```python
from build123d import *

# Parameters (mm, degrees)
CROQUIS1_R              = 0.5
SALIENTE_EXTRUIR1_DEPTH = 3
MATRIZC1_COUNT          = 2
CROQUIS2_R              = 4
CROQUIS2_R_2            = 3
SALIENTE_EXTRUIR2_DEPTH = 2
CHAFL_N1_SIZE           = 1
CHAFL_N1_SIZE2          = 0.577350269


with BuildPart() as part:
    # Croquis1 → Saliente-Extruir1 (new body)
    with BuildSketch(Plane(origin=(0, 0, 0), x_dir=(1, 0, 0), z_dir=(0, 1, 0))):
        with BuildLine():
            Line((-4, 0), (-4, 6.574293681))
            ThreePointArc((-4, 6.574293681), (-3.974394349, 6.996885575), (-3.897952052, 7.413294188))
            Line((-3.897952052, 7.413294188), (-1.698976026, 16.319147094))
            ThreePointArc((-1.698976026, 16.319147094), (0, 17.649646841), (1.698976026, 16.319147094))
            Line((1.698976026, 16.319147094), (3.897952052, 7.413294188))
            ThreePointArc((3.897952052, 7.413294188), (3.974394349, 6.996885575), (4, 6.574293681))
            Line((4, 6.574293681), (4, 0))
            Line((4, 0), (1.25, 0))
            ThreePointArc((1.25, 0), (0, 1.25), (-1.25, 0))
            Line((-1.25, 0), (-4, 0))
        make_face()
        with Locations((0, 15.899646841)):
            Circle(CROQUIS1_R, mode=Mode.SUBTRACT)
        with Locations((0, 12.899646841)):
            Circle(CROQUIS1_R, mode=Mode.SUBTRACT)
        with Locations((0, 9.899646841)):
            Circle(CROQUIS1_R, mode=Mode.SUBTRACT)
        with Locations((0, 6.899646841)):
            Circle(CROQUIS1_R, mode=Mode.SUBTRACT)
    saliente_extruir1 = extrude(amount=SALIENTE_EXTRUIR1_DEPTH)

    # MatrizC1: Saliente-Extruir1 ×2 about axis
    matrizc1_axis = Axis((0, 0, 0), (0, 1, 0))
    for i in range(1, MATRIZC1_COUNT):
        add(saliente_extruir1.rotate(matrizc1_axis, i * 360 / MATRIZC1_COUNT))

    # Croquis2 → Saliente-Extruir2 (add)
    with BuildSketch(Plane(origin=(0, 3, 0), x_dir=(1, 0, 0), z_dir=(0, 1, 0))):
        Circle(CROQUIS2_R)
        Circle(CROQUIS2_R_2, mode=Mode.SUBTRACT)
    extrude(amount=SALIENTE_EXTRUIR2_DEPTH)

    # Chaflán1
    chafl_n1_edges = [part.edges().sort_by_distance(p)[0] for p in [
        (-4, 5, 0),
    ]]
    chafl_n1_side = [part.faces().sort_by_distance(p)[0] for p in [
        (-4, 4, 0),
    ]]
    chamfer(chafl_n1_edges, length=CHAFL_N1_SIZE, length2=CHAFL_N1_SIZE2, reference=chafl_n1_side[0])


solid = part.part
```
Could you check a few things on this model? Use its own coordinates, in mm. A direction names the side the tool comes from. Round coordinates to 2 decimals unless told otherwise and drop trailing zeros. Loops run counter-clockwise (first coordinate to the right, second up) from the corner with the lowest first, then second, coordinate; pieces in that order, holes last.
Q1. I want a section at A-A (y = 2.25). Give the number of separate pieces and of enclosed holes in the cut face, and give its area (3 significant figures).
Q2. Please list where these lines run through material, in increasing order: L1, parallel to Z at x = 0, y = 3.85; L2, parallel to Y at x = -1.75, z = -7; L3, parallel to Z at x = -1, y = 3.2.
Q3. On a 3-axis mill with a long thin cutter (end or side, diameter ignored), from which of +Z, -Z, +X, -X, +Y, -Y can I reach the whole of each face in a straight line? I mean faces 1 (the flat face through (1, 3, -1)), 2 (the flat face through (4, 1, 0)). Say none if no direction works.
Q4. I want a section at D-D (z = -14). Write out the boundary of the cut face in (x, y), and give its area (3 significant figures).
Q5. Thinking about a two-plate mould opening in X: for faces 3 (the cylindrical face through (-0.065, 1.479, -10.395)), 4 (the cylindrical face through (-3.975, 1.479, -6.991)), 5 (the cylindrical face through (-0.03, 1.48, -17.65)), which applies, pulls with the +X half, pulls with the -X half, needs draft (parallel to the pull), parting line crosses it, or undercut?
Q6. For P1, Ø2, axis at y = 2.5, z = -11.5, coming from the +X side; P2, Ø2.5, axis at x = 1.5, z = 11.5, coming from the +Y side; P3, Ø3, axis at y = 3, z = 13.5, coming from the -X side, each with a flat end and sliding along its axis, tell me the tip position at first contact or that it passes through.
Q7. I want a section at C-C (y = 4.7). Write out the boundary of the cut face in (x, z).
Answer below:
1. separate pieces: 1
1. enclosed holes: 9
1. area: 214 mm2
2. L1: z = -4 to -3, 3 to 4
2. L2: y = 0 to 3
2. L3: z = -3.87 to -2.83, 2.83 to 3.87
3. face 1: +Y
3. face 2: +Z, -Z, +X, +Y, -Y
4. outline: (-2.27, 0) - (2.27, 0) - (2.27, 3) - (-2.27, 3) - close
4. area: 13.6 mm2
5. face 3: undercut
5. face 4: pulls with the -X half
5. face 5: parting line crosses it
6. P1: stops at x = 3.14
6. P2: stops at y = 3
6. P3: stops at x = -2.77
7. outline: circle Ø7.19 at (0, 0); hole circle Ø6 at (0, 0)
